Part model, mm, in its own coordinate system. Round coordinates to 2 decimals unless told otherwise and drop trailing zeros. Loops run counter-clockwise (first coordinate to the right, second up) from the corner with the lowest first, then second, coordinate; pieces in that order, holes last.
(1) Mould opens along Z. For faces 1 (the face through (3.472, 31.98, 5.446)), 2 (the face through (0, 32, 8.5)), 3 (the face through (-8.72, 33.94, 0.19)) say: +Z half, -Z half, draft (parallel to the pull), parting line (faces both ways), or undercut.
(2) Cut at A-A on y = 31.4. List the corners of the cut face in (x, z) (1 decimal), then the cut area to 3 significant figures.
(3) Probe probe 1 along Z at (x, y) = (0, 32.65); probe 2 along X at (y, z) = (31.25, -4); probe 3 along Z at (x, y) = (-2.75, 30.6). List the from-to ranges inside material, lowest first.
(4) Flat gauge pin, fed straight in: pin 1 (2 mm diameter, centred on x = 6.5, y = 31.5, fed in from +Z). Where does the tip first touch, or does it go through?
Autodesk Inventor part; units mm, degrees
ref_plane "NUT_TO_BODY_XY" through (0, 30, 0) normal (0, 1, 0) x (1, 0, 0)
ref_plane "NUT_TO_BODY_YZ" through (0, 30, 0) normal (1, 0, 0) x (0, 0, -1)
ref_plane "NUT_TO_BODY_ZX" through (0, 30, 0) normal (0, 0, -1) x (0, 1, 0)
sketch "Sketch_1" plane through (0, 0, 0) normal (0, 0, 1) x (1, 0, 0)
  line L0 (0, 30) -> (0, 34)
  line L1 (0, 34) -> (8.5, 34)
  line L2 (8.5, 34) -> (10.2, 33.5445)
  line L3 (10.2, 33.5445) -> (10.2, 30.4555)
  line L4 (10.2, 30.4555) -> (8.5, 30)
  line L5 (8.5, 30) -> (0, 30)
  line L6 (0, 30) -> (0, 34)
revolve "Revolution1" add sketch "Sketch_1" angle 360 about axis through (0, 30, 0) along (0, -1, 0)
sketch "Sketch_2" plane through (0, 0, 0) normal (0, 0, 1) x (1, 0, 0)
  line L0 (0, 30) -> (0, 34)
  line L1 (0, 34) -> (7, 34)
  line L2 (7, 34) -> (6.4585, 33.4585)
  line L3 (6.4585, 33.4585) -> (6.4585, 30.5415)
  line L4 (6.4585, 30.5415) -> (7, 30)
  line L5 (7, 30) -> (0, 30)
  line L6 (0, 30) -> (0, 34)
revolve "Revolution2" cut sketch "Sketch_2" angle 360 about axis through (0, 30, 0) along (0, -1, 0)
thread "Thread1"
sketch "Sketch_3" plane through (0, 30, 0) normal (0, 1, 0) x (1, 0, 0)
  line L0 (-45, 45) -> (-45, -45)
  line L1 (-45, -45) -> (45, -45)
  line L2 (45, -45) -> (45, 45)
  line L3 (45, 45) -> (-45, 45)
  line L4 (-9.815, 0) -> (-4.9075, -8.5)
  line L5 (-4.9075, -8.5) -> (4.9075, -8.5)
  line L6 (4.9075, -8.5) -> (9.815, 0)
  line L7 (9.815, 0) -> (4.9075, 8.5)
  line L8 (4.9075, 8.5) -> (-4.9075, 8.5)
  line L9 (-4.9075, 8.5) -> (-9.815, 0)
extrude "Extrusion1" cut sketch "Sketch_3" along normal blind 4
ref_plane "NUT_TO_BODY_XY" through (0, 30, 0) normal (0, 1, 0) x (1, 0, 0)
ref_plane "NUT_TO_BODY_YZ" through (0, 30, 0) normal (1, 0, 0) x (0, 0, -1)
ref_plane "NUT_TO_BODY_ZX" through (0, 30, 0) normal (0, 0, -1) x (0, 1, 0)
properties part number "MVFKN40-NUT-NUT"
Final values:
1. face 1: undercut
1. face 2: +Z half
1. face 3: parting line
2. outline: (-9.8, 0) - (-4.9, -8.5) - (4.9, -8.5) - (9.8, 0) - (4.9, 8.5) - (-4.9, 8.5) - close; hole circle Ø12.9 at (0, 0)
2. area: 119 mm2
3. probe 1: z = -8.5 to -6.46, 6.46 to 8.5
3. probe 2: x = -7.51 to -5.07, 5.07 to 7.51
3. probe 3: z = -8.5 to -5.84, 5.84 to 8.5
4. pin 1: stops at z = 7.47
